Here's how the part is built. I have some questions about the finished solid (model axes, mm). Face numbers are marked on the shaded views. A direction names the side the tool comes from. Round coordinates to 2 decimals unless told otherwise and drop trailing zeros. Loops run counter-clockwise (first coordinate to the right, second up) from the corner with the lowest first, then second, coordinate; pieces in that order, holes last. Notation, with made-up numbers: M -3.5,65.5 L 12.5,65.5 A14 cw 12.5,77.5 Z; hole C 4,58.25 d1. An arc over 180 degrees is marked long. Answer as a JSON object with one key per item and string values.
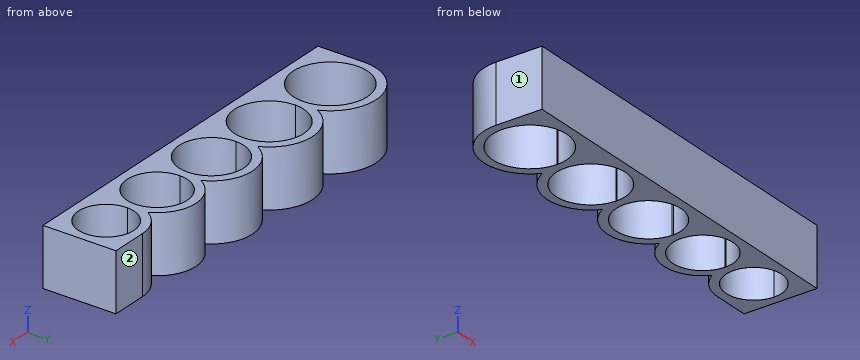
from build123d import *

# Parameters (mm, degrees)
F1_DEPTH = 25.4


with BuildPart() as f1:
    # F0 (on Top) → F1 (new body)
    with BuildSketch(Plane.XY):
        with BuildLine():
            ThreePointArc((0, 0), (-14.1888046713, 5.8771953287), (-20.066, 20.066))
            Line((-20.066, 20.066), (-20.066, 0))
            Line((-20.066, 0), (0, 0))
        make_face()
        with BuildLine():
            ThreePointArc((17.9660905129, 11.129336882), (16.6211524445, 15.2651396685), (16.2492676931, 19.598201499))
            ThreePointArc((16.2492676931, 19.598201499), (16.8698181027, 23.9026921501), (18.4504618661, 27.9542705917))
            ThreePointArc((18.4504618661, 27.9542705917), (-4.0260022476, 39.7239668812), (-20.066, 20.066))
            ThreePointArc((-20.066, 20.066), (-14.1888046713, 5.8771953287), (0, 0))
            ThreePointArc((0, 0), (10.5669596828, 3.0077551002), (17.9660905129, 11.129336882))
        make_face()
        with BuildLine():
            ThreePointArc((16.2492676931, 19.598201499), (-16.2543168361, 20.2999234712), (16.256, 20.066))
            ThreePointArc((16.256, 20.066), (16.2543168361, 19.8320765288), (16.2492676931, 19.598201499))
        make_face(mode=Mode.SUBTRACT)
        with BuildLine():
            ThreePointArc((18.4504618661, 27.9542705917), (16.8698181027, 23.9026921501), (16.2492676931, 19.598201499))
            ThreePointArc((16.2492676931, 19.598201499), (16.6211524445, 15.2651396685), (17.9660905129, 11.129336882))
            ThreePointArc((17.9660905129, 11.129336882), (19.4658964939, 15.1953501781), (20.0576898143, 19.4885614204))
            ThreePointArc((20.0576898143, 19.4885614204), (20.063922346, 19.7772508128), (20.066, 20.066))
            ThreePointArc((20.066, 20.066), (19.6579668812, 24.0920022476), (18.4504618661, 27.9542705917))
        make_face()
        with BuildLine():
            ThreePointArc((35.2913783636, 0), (24.9954114371, 3.0220379638), (17.9660905129, 11.129336882))
            ThreePointArc((17.9660905129, 11.129336882), (10.5669596828, 3.0077551002), (0, 0))
            Line((0, 0), (35.2913783636, 0))
        make_face()
        with BuildLine():
            ThreePointArc((52.7363723922, 26.7034096963), (35.9859218001, 38.087334616), (18.4504618661, 27.9542705917))
            ThreePointArc((18.4504618661, 27.9542705917), (19.6579668812, 24.0920022476), (20.066, 20.066))
            ThreePointArc((20.066, 20.066), (20.063922346, 19.7772508128), (20.0576898143, 19.4885614204))
            ThreePointArc((20.0576898143, 19.4885614204), (35.5106816843, 34.2884220315), (50.5313782672, 19.05))
            ThreePointArc((50.5313782672, 19.05), (50.5296016293, 18.8173011199), (50.5242721296, 18.5846564946))
            ThreePointArc((50.5242721296, 18.5846564946), (51.150167686, 22.7748598412), (52.7363723922, 26.7034096963))
        make_face()
        with BuildLine():
            ThreePointArc((20.0576898143, 19.4885614204), (19.4658964939, 15.1953501781), (17.9660905129, 11.129336882))
            ThreePointArc((17.9660905129, 11.129336882), (24.9954114371, 3.0220379638), (35.2913783636, 0))
            ThreePointArc((35.2913783636, 0), (45.2184017505, 2.7909500658), (52.2366769647, 10.3460151624))
            ThreePointArc((52.2366769647, 10.3460151624), (50.8932296176, 14.3640617786), (50.5242721296, 18.5846564946))
            ThreePointArc((50.5242721296, 18.5846564946), (34.8394256297, 3.8167029566), (20.0576898143, 19.4885614204))
        make_face()
        with BuildLine():
            ThreePointArc((54.3413782672, 19.05), (53.9358095817, 22.9599464139), (52.7363723922, 26.7034096963))
            ThreePointArc((52.7363723922, 26.7034096963), (51.150167686, 22.7748598412), (50.5242721296, 18.5846564946))
            ThreePointArc((50.5242721296, 18.5846564946), (50.8932296176, 14.3640617786), (52.2366769647, 10.3460151624))
            ThreePointArc((52.2366769647, 10.3460151624), (53.7372042015, 14.2903775777), (54.3324955841, 18.4683202558))
            ThreePointArc((54.3324955841, 18.4683202558), (54.339157467, 18.7591262186), (54.3413782672, 19.05))
        make_face()
        with BuildLine():
            ThreePointArc((52.2366769647, 10.3460151624), (45.2184017505, 2.7909500658), (35.2913783636, 0))
            Line((35.2913783636, 0), (68.5498631996, 0))
            ThreePointArc((68.5498631996, 0), (58.8911873733, 2.8045831602), (52.2366769647, 10.3460151624))
        make_face()
        with BuildLine():
            ThreePointArc((54.3324955841, 18.4683202558), (53.7372042015, 14.2903775777), (52.2366769647, 10.3460151624))
            ThreePointArc((52.2366769647, 10.3460151624), (58.8911873733, 2.8045831602), (68.5498631996, 0))
            ThreePointArc((68.5498631996, 0), (77.8389985645, 2.576408979), (84.4739682688, 9.5694838446))
            ThreePointArc((84.4739682688, 9.5694838446), (83.1320884093, 13.4663031835), (82.7663397489, 17.5714305184))
            ThreePointArc((82.7663397489, 17.5714305184), (68.1014181096, 3.8170709012), (54.3324955841, 18.4683202558))
        make_face()
        with BuildLine():
            ThreePointArc((86.5838631996, 18.034), (86.1810315428, 21.8243903304), (84.9905329505, 25.4454461574))
            ThreePointArc((84.9905329505, 25.4454461574), (83.3981736494, 21.644099363), (82.7663397489, 17.5714305184))
            ThreePointArc((82.7663397489, 17.5714305184), (83.1320884093, 13.4663031835), (84.4739682688, 9.5694838446))
            ThreePointArc((84.4739682688, 9.5694838446), (85.9751949602, 13.388252586), (86.5743245521, 17.4475283849))
            ThreePointArc((86.5743245521, 17.4475283849), (86.5814783801, 17.7407254097), (86.5838631996, 18.034))
        make_face()
        with BuildLine():
            ThreePointArc((84.9905329505, 25.4454461574), (69.2526835345, 36.0542996528), (52.7363723922, 26.7034096963))
            ThreePointArc((52.7363723922, 26.7034096963), (53.9358095817, 22.9599464139), (54.3413782672, 19.05))
            ThreePointArc((54.3413782672, 19.05), (54.339157467, 18.7591262186), (54.3324955841, 18.4683202558))
            ThreePointArc((54.3324955841, 18.4683202558), (68.7670486464, 32.2563418072), (82.7738631996, 18.034))
            ThreePointArc((82.7738631996, 18.034), (82.7719822126, 17.80268467), (82.7663397489, 17.5714305184))
            ThreePointArc((82.7663397489, 17.5714305184), (83.3981736494, 21.644099363), (84.9905329505, 25.4454461574))
        make_face()
        with BuildLine():
            ThreePointArc((84.4739682688, 9.5694838446), (77.8389985645, 2.576408979), (68.5498631996, 0))
            Line((68.5498631996, 0), (99.7753385043, 0))
            ThreePointArc((99.7753385043, 0), (90.751661979, 2.5893622969), (84.4739682688, 9.5694838446))
        make_face()
        with BuildLine():
            ThreePointArc((86.5743245521, 17.4475283849), (85.9751949602, 13.388252586), (84.4739682688, 9.5694838446))
            ThreePointArc((84.4739682688, 9.5694838446), (90.751661979, 2.5893622969), (99.7753385043, 0))
            ThreePointArc((99.7753385043, 0), (108.4287993719, 2.3643335983), (114.6777863565, 8.8003743081))
            ThreePointArc((114.6777863565, 8.8003743081), (113.3375545812, 12.572175467), (112.9753463662, 16.5585912009))
            ThreePointArc((112.9753463662, 16.5585912009), (99.3308696276, 3.8174806383), (86.5743245521, 17.4475283849))
        make_face()
        with BuildLine():
            ThreePointArc((115.2130425103, 24.1796771097), (100.4874564143, 34.0210941914), (84.9905329505, 25.4454461574))
            ThreePointArc((84.9905329505, 25.4454461574), (86.1810315428, 21.8243903304), (86.5838631996, 18.034))
            ThreePointArc((86.5838631996, 18.034), (86.5814783801, 17.7407254097), (86.5743245521, 17.4475283849))
            ThreePointArc((86.5743245521, 17.4475283849), (99.9901311009, 30.2242533726), (112.9833385043, 17.018))
            ThreePointArc((112.9833385043, 17.018), (112.9813403186, 16.7882608441), (112.9753463662, 16.5585912009))
            ThreePointArc((112.9753463662, 16.5585912009), (113.6138262125, 20.5101794262), (115.2130425103, 24.1796771097))
        make_face()
        with BuildLine():
            ThreePointArc((116.7933385043, 17.018), (116.3935690174, 20.6849794945), (115.2130425103, 24.1796771097))
            ThreePointArc((115.2130425103, 24.1796771097), (113.6138262125, 20.5101794262), (112.9753463662, 16.5585912009))
            ThreePointArc((112.9753463662, 16.5585912009), (113.3375545812, 12.572175467), (114.6777863565, 8.8003743081))
            ThreePointArc((114.6777863565, 8.8003743081), (116.1796742164, 12.4891928897), (116.7830409477, 16.4260696034))
            ThreePointArc((116.7830409477, 16.4260696034), (116.7907639204, 16.7219900196), (116.7933385043, 17.018))
        make_face()
        with BuildLine():
            ThreePointArc((128.9676635915, 32.004), (121.0554952765, 29.9110472914), (115.2130425103, 24.1796771097))
            ThreePointArc((115.2130425103, 24.1796771097), (116.3935690174, 20.6849794945), (116.7933385043, 17.018))
            ThreePointArc((116.7933385043, 17.018), (116.7907639204, 16.7219900196), (116.7830409477, 16.4260696034))
            ThreePointArc((116.7830409477, 16.4260696034), (116.1796742164, 12.4891928897), (114.6777863565, 8.8003743081))
            ThreePointArc((114.6777863565, 8.8003743081), (120.5764899645, 2.3765748998), (128.9676635915, 0))
            ThreePointArc((128.9676635915, 0), (140.2827863041, 4.6868772875), (144.9696635915, 16.002))
            ThreePointArc((144.9696635915, 16.002), (140.2827863041, 27.3171227125), (128.9676635915, 32.004))
        make_face()
        with BuildLine():
            ThreePointArc((141.1596635915, 16.002), (128.7555967071, 3.8118444786), (116.7830409477, 16.4260696034))
            ThreePointArc((116.7830409477, 16.4260696034), (129.179730476, 28.1921555214), (141.1596635915, 16.002))
        make_face(mode=Mode.SUBTRACT)
        with BuildLine():
            ThreePointArc((114.6777863565, 8.8003743081), (108.4287993719, 2.3643335983), (99.7753385043, 0))
            Line((99.7753385043, 0), (128.9676635915, 0))
            ThreePointArc((128.9676635915, 0), (120.5764899645, 2.3765748998), (114.6777863565, 8.8003743081))
        make_face()
        with BuildLine():
            ThreePointArc((144.9696635915, 16.002), (140.2827863041, 4.6868772875), (128.9676635915, 0))
            Line((128.9676635915, 0), (144.9696635915, 0))
            Line((144.9696635915, 0), (144.9696635915, 16.002))
        make_face()
        with BuildLine():
            Line((144.9696635915, 32.004), (128.9676635915, 32.004))
            ThreePointArc((128.9676635915, 32.004), (140.2827863041, 27.3171227125), (144.9696635915, 16.002))
            Line((144.9696635915, 16.002), (144.9696635915, 32.004))
        make_face()
    extrude(amount=F1_DEPTH)


solid = f1.part
Item 1: I want a section at B-B on y = 10. List the corners of the cut face in (x, z) for me.
Solution:
{"outline": "M -20.07,0 L -12.76,0 L -12.76,25.4 L -20.07,25.4 Z; M 12.76,0 L 23.03,0 L 23.03,25.4 L 12.76,25.4 Z; M 47.55,0 L 56.81,0 L 56.81,25.4 L 47.55,25.4 Z; M 80.29,0 L 88.59,0 L 88.59,25.4 L 80.29,25.4 Z; M 110.96,0 L 118.36,0 L 118.36,25.4 L 110.96,25.4 Z; M 139.58,0 L 144.97,0 L 144.97,25.4 L 139.58,25.4 Z"}
Item 2: I want a section at A-A on x = 0. List the corners of the cut face in (y, z) for me.
Solution:
{"outline": "M 0,0 L 3.81,0 L 3.81,25.4 L 0,25.4 Z; M 36.32,0 L 40.13,0 L 40.13,25.4 L 36.32,25.4 Z"}
Item 3: For P1, Ø5, axis at x = 120, z = 11, coming from the +Y side; P2, Ø3, axis at y = 36, z = 11, coming from the -X side; P3, Ø2, axis at x = 28.5, z = 13.5, coming from the -Y side; P4, Ø4, axis at x = 48, y = 36, coming from the +Z side, each with a flat end and sliding along its axis, tell me the tip position at first contact or that it passes through.
Solution:
{"P1": "stops at y = 30.64", "P2": "stops at x = -13.94", "P3": "stops at y = 0", "P4": "passes through"}
Item 4: I want a section at D-D on x = 35. List the corners of the cut face in (y, z) for me, plus the area to 3 significant figures.
Solution:
{"outline": "M 0,0 L 3.81,0 L 3.81,25.4 L 0,25.4 Z; M 34.29,0 L 38.1,0 L 38.1,25.4 L 34.29,25.4 Z", "area": "194 mm2"}
Item 5: I want a section at C-C on z = 15.5. List the corners of the cut face in (x, y) for me.
Solution:
{"outline": "M -20.07,0 L 144.97,0 L 144.97,32 L 128.97,32 A16 ccw 115.21,24.18 A17.02 ccw 84.99,25.45 A18.03 ccw 52.74,26.7 A19.05 ccw 18.45,27.95 A20.07 ccw -20.07,20.07 Z; hole C 0,20.07 d32.51; hole C 35.29,19.05 d30.48; hole C 68.55,18.03 d28.45; hole C 99.78,17.02 d26.42; hole C 128.97,16 d24.38"}
Item 6: For the marked faces 1 and 2, which set-ups out of +Z, -Z, +X, -X, +Y, -Y let a thin tool reach every point of the face, with its end or its side?
Solution:
{"face 1": "+Z, -Z, -X, +Y, -Y", "face 2": "+Z, -Z, +X, +Y"}
Item 7: If I drill on L1, parallel to Y at x = 0, z = 12.5; L2, parallel to X at y = 9, z = 1.5; L3, parallel to X at y = 13, z = 23.75, over which ranges is the centre line in solid material (lowest first)? Write a range as from..to.
Solution:
{"L1": "y = 0..3.81, 36.32..40.13", "L2": "x = -20.07..-11.91, 11.91..23.83, 46.75..57.56, 79.54..89.28, 110.27..118.99, 138.95..144.97", "L3": "x = -20.07..-14.64, 14.64..21.3, 49.28..55.25, 81.85..87.19, 112.36..117.15, 140.78..144.97"}
